```python
from build123d import *

# Parameters (mm, degrees)
PAD_DEPTH       = 22
SKETCH001_W     = 13.45
SKETCH001_H     = 13.45
POCKET_DEPTH    = 20
SKETCH002_W     = 13.45
SKETCH002_H     = 13.45
POCKET001_DEPTH = 20
POCKET002_DEPTH = 5
CHAMFER_SIZE    = 2
FILLET_R        = 5


with BuildPart() as part:
    # Sketch → Pad (new body)
    with BuildSketch(Plane.XY):
        Polygon((-11, 24.556349), (11, 24.556349), (11, 4.556349), (25.142136, -9.585786), (9.585786, -25.142136), (-11, -4.556349), align=None)
    extrude(amount=PAD_DEPTH)

    # Sketch001 (on Face4 of Pad) → Pocket (cut)
    with BuildSketch(Plane(origin=(17.363961, -17.363961, 0), x_dir=(0.707107, 0.707107, 0), z_dir=(0.707107, -0.707107, 0))):
        with Locations((0, 11)):
            Rectangle(SKETCH001_W, SKETCH001_H)
    extrude(amount=-POCKET_DEPTH, mode=Mode.SUBTRACT)

    # Sketch002 (on Face1 of Pocket) → Pocket001 (cut)
    with BuildSketch(Plane(origin=(0, 24.556349, 0), x_dir=(-1, 0, 0), z_dir=(0, 1, 0))):
        with Locations((0, 11)):
            Rectangle(SKETCH002_W, SKETCH002_H)
    extrude(amount=-POCKET001_DEPTH, mode=Mode.SUBTRACT)

    # Sketch003 (on Face3 of Pocket001) → Pocket002 (cut)
    with BuildSketch(Plane(origin=(0, 0, 0), x_dir=(1, 0, 0), z_dir=(0, 0, -1))):
        with BuildLine():
            ThreePointArc((1.7, -10.528175), (0, -8.828175), (-1.7, -10.528175))
            Line((-1.7, -10.528175), (-1.7, -14.028175))
            ThreePointArc((-1.7, -14.028175), (0, -15.728175), (1.7, -14.028175))
            Line((1.7, -10.528175), (1.7, -14.028175))
        make_face()
        with BuildLine():
            Line((8.717336, 11.121499), (6.242462, 8.646625))
            ThreePointArc((6.242462, 8.646625), (6.242462, 6.242462), (8.646625, 6.242462))
            Line((11.121499, 8.717336), (8.646625, 6.242462))
            ThreePointArc((11.121499, 8.717336), (11.121499, 11.121499), (8.717336, 11.121499))
        make_face()
    extrude(amount=-POCKET002_DEPTH, mode=Mode.SUBTRACT)

    # Chamfer
    chamfer_edges = [part.edges().sort_by_distance(p)[0] for p in [
        (9.884062, -7.479899, 0),
        (11.121499, -11.121499, 0),
        (7.479899, -9.884062, 0),
        (6.242462, -6.242462, 0),
        (0, 8.828175, 0),
        (1.7, 12.278175, 0),
        (0, 15.728175, 0),
        (-1.7, 12.278175, 0),
    ]]
    chamfer(chamfer_edges, length=CHAMFER_SIZE)

    # Fillet
    fillet_edges = [part.edges().sort_by_distance(p)[0] for p in [
        (-11, -4.556349, 11),
        (11, 4.556349, 11),
    ]]
    fillet(fillet_edges, radius=FILLET_R)


solid = part.part
```
Geometry: final body of the model. Coordinates: model frame, mm. A direction names the side the tool comes from. Round coordinates to 2 decimals unless told otherwise and drop trailing zeros. Write each loop counter-clockwise with the first axis right and the second up, starting at its lowest first coordinate (ties: lowest second). Pieces come first, ordered by that corner, then holes.
Item 1: Section query B-B (z = 10.75). Return loops of the section in (x, y) (3 decimals), plus the area to 3 significant figures.
Item 2: Section query C-C (y = 13). Return loops of the section in (x, z) (3 decimals).
Item 3: Material intervals for L1, parallel to X at y = 8, z = 13 (3 decimals); L2, parallel to Z at x = -0.5, y = 6.5 (3 decimals); L3, parallel to Y at x = 7.5, z = 8.75, sorted ascending.
Item 4: Section query A-A (x = 0). Return loops of the section in (y, z) (3 decimals), plus the area to 3 significant figures.
Item 5: Pin query (flat end, axial travel): P1, Ø6, axis at x = 7.5, y = -4, coming from the -Z side; P2, Ø2, axis at y = -19.5, z = 16, coming from the -X side; P3, Ø4, axis at x = 0, z = 9, coming from the +Y side; P4, Ø11, axis at y = 14.5, z = 13, coming from the +X side. Return the tip coordinate at first contact, or that it passes through.
Item 6: Mould query, pull axis X, two halves, no side actions, for faces 5 (the face through (7.497, -9.901, 3.122)), 6 (the face through (3, 0, 22)), 7 (the face through (11, 16, 11)), 8 (the face through (-6.725, 15, 11)). Classes: +X half, -X half, draft (parallel to the pull), parting line (faces both ways), or undercut.
Item 7: Section query D-D (x = 19.5). Return loops of the section in (y, z) (3 decimals), plus the area to 3 significant figures.
Item 8: Set-up query: faces 1 (the face through (6.725, 15, 11)), 2 (the face through (6.216, -6.269, 3.122)), 3 (the face through (18.715, -3.158, 10.846)), 4 (the face through (5.64, -15.15, 10.91)). Return all of +Z, -Z, +X, -X, +Y, -Y with unobstructed straight access to the full face (end or side cutting, diameter ignored); none if empty.
Completed:
1. outline: (-11, -2.485) arc R5 ccw to (-9.536, -6.021) - (9.586, -25.142) - (12.609, -22.119) - (-1.533, -7.977) - (7.977, 1.533) - (22.119, -12.609) - (25.142, -9.586) - (12.464, 3.092) arc R5 cw to (11, 6.627) - (11, 24.556) - (6.725, 24.556) - (6.725, 4.556) - (-6.725, 4.556) - (-6.725, 24.556) - (-11, 24.556) - close
1. area: 542 mm2
2. outline: (-11, 0) - (-3.7, 0) - (-1.7, 2) - (-1.7, 4.275) - (-6.725, 4.275) - (-6.725, 17.725) - (6.725, 17.725) - (6.725, 4.275) - (1.7, 4.275) - (1.7, 2) - (3.7, 0) - (11, 0) - (11, 22) - (-11, 22) - close
3. L1: x = -11 to -6.725, 6.725 to 11
3. L2: z = 0 to 4.275, 17.725 to 22
3. L3: y = -23.06 to -17.01, 1.06 to 24.56
4. outline: (-15.556, 0) - (6.828, 0) - (8.828, 2) - (8.828, 4.275) - (4.556, 4.275) - (4.556, 17.725) - (24.556, 17.725) - (24.556, 22) - (-15.556, 22) - close; (15.728, 2) - (17.728, 0) - (24.556, 0) - (24.556, 4.275) - (15.728, 4.275) - close; hole (-9.511, 4.275) - (-6.444, 4.275) - (-6.444, 17.725) - (-9.511, 17.725) - close
4. area: 539 mm2
5. P1: stops at z = 0
5. P2: stops at x = 2.94
5. P3: stops at y = 4.56
5. P4: stops at x = 11
6. face 5: undercut
6. face 6: draft
6. face 7: +X half
6. face 8: undercut
7. outline: (-15.228, 0) - (-3.944, 0) - (-3.944, 22) - (-15.228, 22) - (-15.228, 17.725) - (-9.989, 17.725) - (-9.989, 4.275) - (-15.228, 4.275) - close
7. area: 178 mm2
8. face 1: +Y
8. face 2: -Z
8. face 3: +Z, -Z, +X, +Y
8. face 4: none
